from build123d import *

# Parameters (mm, degrees)
BOSS_EXTRUDE1_DEPTH                             = 4.75
BOSS_EXTRUDE1_DEPTH_BACK                        = 15.25
SKETCH1_W                                       = 150
SKETCH1_H                                       = 85
SKETCH2_R                                       = 21.5
F_1MM_CLEARANCE_DEPTH                           = 12
SKETCH5_R                                       = 41
CUT_EXTRUDE2_DEPTH                              = 3.5
SKETCH6_R                                       = 14
CUT_EXTRUDE3_DEPTH                              = 11.5
CSK_FOR_M8_FLAT_HEAD_MACHINE_SCREW1_D           = 9
CSK_FOR_M8_FLAT_HEAD_MACHINE_SCREW1_CSINK_D     = 17.3
CSK_FOR_M8_FLAT_HEAD_MACHINE_SCREW1_CSINK_ANGLE = 90
CSK_FOR_M4_FLAT_HEAD_MACHINE_SCREW1_D           = 4.5
CSK_FOR_M4_FLAT_HEAD_MACHINE_SCREW1_CSINK_D     = 9.4
CSK_FOR_M4_FLAT_HEAD_MACHINE_SCREW1_CSINK_ANGLE = 90
M4X0_7_TAPPED_HOLE1_D                           = 3.3
M4X0_7_TAPPED_HOLE1_DEPTH                       = 10.1
M4X0_7_TAPPED_HOLE1_TIP                         = 0.991420021


with BuildPart() as part:
    # Sketch1 → Boss-Extrude1 (new, two sides: drawn at the far end of the back side and taken through both)
    with BuildSketch(Plane.ZY.offset(-152.244801117).offset(-BOSS_EXTRUDE1_DEPTH_BACK)):
        with Locations((-933.40139902, 151.879264394)):
            Rectangle(SKETCH1_W, SKETCH1_H)
    extrude(amount=BOSS_EXTRUDE1_DEPTH + BOSS_EXTRUDE1_DEPTH_BACK)

    # Sketch2 → 1mm clearance (cut)
    with BuildSketch(Plane(origin=(167.494801117, 0, 0), x_dir=(0, 0, -1), z_dir=(1, 0, 0))):
        with Locations((933.40139902, 151.879264394)):
            Circle(SKETCH2_R)
    extrude(amount=-F_1MM_CLEARANCE_DEPTH, mode=Mode.SUBTRACT)

    # Sketch5 → Cut-Extrude2 (cut)
    with BuildSketch(Plane.ZY.offset(-147.494801117)):
        with Locations((-933.40139902, 151.879264394)):
            Circle(SKETCH5_R)
    extrude(amount=-CUT_EXTRUDE2_DEPTH, mode=Mode.SUBTRACT)

    # Sketch6 → Cut-Extrude3 (cut)
    with BuildSketch(Plane.ZY.offset(-150.994801117)):
        with Locations((-933.40139902, 151.879264394)):
            Circle(SKETCH6_R)
    extrude(amount=-CUT_EXTRUDE3_DEPTH, mode=Mode.SUBTRACT)

    # CSK for M8 Flat Head Machine Screw1 (through all)
    with Locations(Plane.ZY.offset(-147.494801117)):
        with Locations((-878.40139902, 129.379264394), (-878.40139902, 174.379264394), (-988.40139902, 129.379264394), (-988.40139902, 174.379264394)):
            CounterSinkHole(CSK_FOR_M8_FLAT_HEAD_MACHINE_SCREW1_D / 2, CSK_FOR_M8_FLAT_HEAD_MACHINE_SCREW1_CSINK_D / 2, counter_sink_angle=CSK_FOR_M8_FLAT_HEAD_MACHINE_SCREW1_CSINK_ANGLE)

    # CSK for M4 Flat Head Machine Screw1 (through all)
    with Locations(Plane.ZY.offset(-150.994801117)):
        with Locations((-933.40139902, 134.379264394), (-950.90139902, 151.879264394), (-915.90139902, 151.879264394), (-933.40139902, 169.379264394)):
            CounterSinkHole(CSK_FOR_M4_FLAT_HEAD_MACHINE_SCREW1_D / 2, CSK_FOR_M4_FLAT_HEAD_MACHINE_SCREW1_CSINK_D / 2, counter_sink_angle=CSK_FOR_M4_FLAT_HEAD_MACHINE_SCREW1_CSINK_ANGLE)

    # M4x0.7 Tapped Hole1
    with Locations(Plane.ZY.offset(-147.494801117)):
        with Locations((-878.40139902, 151.879264394), (-973.40139902, 121.879264394), (-973.40139902, 181.879264394)):
            Hole(M4X0_7_TAPPED_HOLE1_D / 2, depth=M4X0_7_TAPPED_HOLE1_DEPTH)
            with Locations((0, 0, -(M4X0_7_TAPPED_HOLE1_DEPTH + M4X0_7_TAPPED_HOLE1_TIP / 2))):  # 118° drill point
                Cone(0, M4X0_7_TAPPED_HOLE1_D / 2, M4X0_7_TAPPED_HOLE1_TIP, mode=Mode.SUBTRACT)


solid = part.part
For this review, take the finished solid that the model builds, in its own axes (mm). A direction names the side the tool comes from. Give positions to 0.01 mm unless a question says otherwise; leave off trailing zeros. Order: outer loops, then holes, each group sorted by start corner. A loop starts at its lowest first (then second) coordinate and runs counter-clockwise, first axis right, second up. Notation, with made-up numbers: (44, -12) -> (73, -12) arc R28 ccw to (73, 11) -> close; hole circle Ø1 at (18, 69.5). An arc over 180 degrees is marked (long way). Write item = value, one per line.
1) To check wall thickness, follow L1, parallel to Z at x = 160.5, y = 151; L2, parallel to Z at x = 163, y = 178.5; L3, parallel to Z at x = 153, y = 132.5. State the ranges of each line that lie inside material, in increasing order. Write a range as from..to.
Findings:
L1 = -1008.4..-954.88, -911.92..-858.4
L2 = -1008.4..-990.21, -986.59..-880.21, -876.59..-858.4
L3 = -1008.4..-991.64, -985.16..-935.33, -931.47..-881.64, -875.16..-858.4
2) We need section B-B, the plane x = 161. Give the boundary of the cut face in (y, z).
Findings:
outline = (109.38, -1008.4) -> (194.38, -1008.4) -> (194.38, -858.4) -> (109.38, -858.4) -> close; hole circle Ø9 at (129.38, -988.4); hole circle Ø9 at (129.38, -878.4); hole circle Ø43 at (151.88, -933.4); hole circle Ø9 at (174.38, -988.4); hole circle Ø9 at (174.38, -878.4)
3) Insertion check: pin 1 (6 mm diameter, centred on y = 151.88, z = -950.9, fed in from -X); pin 2 (4 mm diameter, centred on y = 169.38, z = -933.4, fed in from +X); pin 3 (3 mm diameter, centred on y = 181.88, z = -973.4, fed in from -X); pin 4 (8 mm diameter, centred on y = 181.5, z = -930, fed in from -X). Each pin has a flat end and moves straight along its axis. Give the tip position at first contact, or say it passes through.
Findings:
pin_1 = 152.69
pin_2 = through
pin_3 = 157.68
pin_4 = 150.99
4) For faces 5 (the face through (154.484, 151.978, -948.654)), 6 (the face through (155.495, 138, -938)), 7 (the face through (149.22, 179.59, -963.62)), list the 3-axis set-ups (+Z, -Z, +X, -X, +Y, -Y) from which the entire face can be reached by the end or side of a thin tool; tool diameter is ignored.
Findings:
face_5 = +X, -X
face_6 = +X
face_7 = -X
5) We need section D-D, the plane y = 117. Give the boundary of the cut face in (x, z).
Findings:
outline = (147.49, -1008.4) -> (167.49, -1008.4) -> (167.49, -858.4) -> (147.49, -858.4) -> (147.49, -911.85) -> (150.99, -911.85) -> (150.99, -954.95) -> (147.49, -954.95) -> close
6) Draft analysis for pull direction Z (two halves, no side actions). For faces 1 (the face through (158, 109.379, -934)), 2 (the face through (158, 151, -1008.401)), 3 (the face through (158, 151, -858.401)), 4 (the face through (154.484, 169.478, -931.154)), state which applies: pulls with the +Z half, pulls with the -Z half, needs draft (parallel to the pull), parting line crosses it, or undercut.
Findings:
face_1 = needs draft
face_2 = pulls with the -Z half
face_3 = pulls with the +Z half
face_4 = undercut
7) We need section A-A, the plane y = 144. Give the boundary of the cut face in (x, z).
Findings:
outline = (147.49, -1008.4) -> (167.49, -1008.4) -> (167.49, -953.41) -> (155.49, -953.41) -> (155.49, -944.97) -> (150.99, -944.97) -> (150.99, -973.64) -> (147.49, -973.64) -> close; (147.49, -893.17) -> (150.99, -893.17) -> (150.99, -921.83) -> (155.49, -921.83) -> (155.49, -913.4) -> (167.49, -913.4) -> (167.49, -858.4) -> (147.49, -858.4) -> close
8) We need section C-C, the plane z = -904.5. Give the boundary of the cut face in (x, y).
Findings:
outline = (147.49, 109.38) -> (167.49, 109.38) -> (167.49, 194.38) -> (147.49, 194.38) -> (147.49, 180.96) -> (150.99, 180.96) -> (150.99, 122.8) -> (147.49, 122.8) -> close
